Here's how the part is built. I have some questions about the finished solid (model axes, mm). Face numbers are marked on the shaded views. A direction names the side the tool comes from. Round coordinates to 2 decimals unless told otherwise and drop trailing zeros. Write each loop counter-clockwise with the first axis right and the second up, starting at its lowest first coordinate (ties: lowest second). Pieces come first, ordered by that corner, then holes. Notation, with made-up numbers: M 31.5,54 L 39.5,54 A16 ccw 39.5,78 Z; hole C 28,4 d4. An arc over 180 degrees is marked long. Use a Markdown table: item, result. Add a question column.
```python
from build123d import *

# Parameters (mm, degrees)
SKETCH1_R           = 1.5
BOSS_EXTRUDE1_DEPTH = 3


with BuildPart() as part:
    # Sketch1 → Boss-Extrude1 (new body)
    with BuildSketch(Plane.XY):
        with BuildLine():
            Line((0, 7), (0, 12))
            Line((0, 12), (3, 12))
            Line((3, 12), (3, 16))
            Line((3, 16), (0, 16))
            Line((0, 16), (0, 21))
            Line((0, 21), (3, 21))
            Line((3, 21), (3, 25))
            Line((3, 25), (0, 25))
            Line((0, 25), (0, 30))
            Line((0, 30), (3, 30))
            Line((3, 30), (3, 34))
            Line((3, 34), (0, 34))
            Line((0, 34), (0, 39))
            Line((0, 39), (3, 39))
            Line((3, 39), (3, 43))
            Line((3, 43), (0, 43))
            Line((0, 43), (0, 48))
            Line((0, 48), (3, 48))
            Line((3, 48), (3, 52))
            Line((3, 52), (0, 52))
            Line((0, 52), (0, 57))
            Line((0, 57), (3, 57))
            Line((3, 57), (3, 61))
            Line((3, 61), (0, 61))
            Line((0, 61), (0, 66))
            Line((0, 66), (3, 66))
            Line((3, 66), (3, 70))
            Line((3, 70), (0, 70))
            Line((0, 70), (0, 75))
            Line((0, 75), (3, 75))
            Line((3, 75), (3, 79))
            Line((3, 79), (0, 79))
            Line((0, 79), (0, 84))
            Line((0, 84), (2, 84))
            ThreePointArc((2, 84), (4.121320344, 83.121320344), (5, 81))
            Line((5, 81), (5, 59.197256694))
            ThreePointArc((5, 59.197256694), (5.006464082, 59.000425028), (5.02582847, 58.804441586))
            Line((5.02582847, 58.804441586), (12, 6))
            Line((12, 6), (12, 4))
            ThreePointArc((12, 4), (10.828427125, 1.171572875), (8, 0))
            Line((8, 0), (0, 0))
            Line((0, 0), (0, 3))
            Line((0, 3), (3, 3))
            Line((3, 3), (3, 7))
            Line((3, 7), (0, 7))
        make_face()
        with Locations((8, 5)):
            Circle(SKETCH1_R, mode=Mode.SUBTRACT)
    extrude(amount=BOSS_EXTRUDE1_DEPTH)


solid = part.part
```
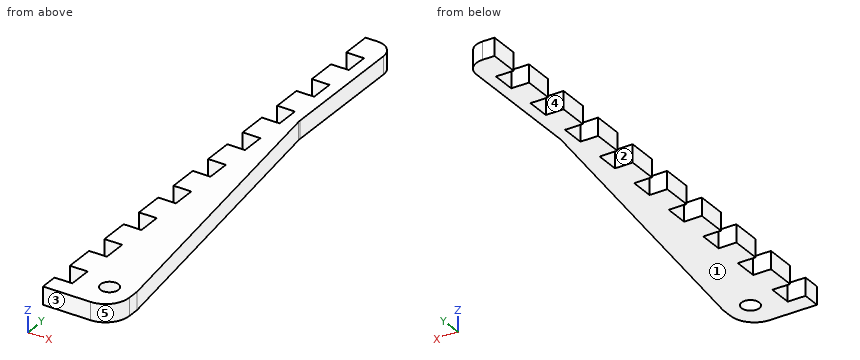
Item 1: If we mould it in two halves opening along Y, with no side actions, what happens to the marked faces 1, 2 and 3? For each: +Y half, -Y half, draft (parallel to the pull), parting line (faces both ways), or undercut.
Item 2: Imagine slicing it at B-B on x = 8.75. List the corners of the cut face in (y, z) for me.
Item 3: Imagine slicing it at A-A on y = 5. List the corners of the cut face in (x, z) for me, plus the area to 3 significant figures.
Item 4: I need wall thicknesses on probe 1 along X at (y, z) = (59, 2.45); probe 2 along X at (y, z) = (4.5, 0.6); probe 3 along X at (y, z) = (43.5, 2.85). Which ranges of each line are inside material? Lowest first, please. Write a range as from..to.
Item 5: On a 3-axis mill with a long thin cutter (end or side, diameter ignored), from which of +Z, -Z, +X, -X, +Y, -Y can I reach the whole of each face in a straight line? I mean the marked faces 4 and 5. Say none if no direction works.
Item 6: Imagine slicing it at C-C on y = 28. List the corners of the cut face in (x, z) for me.
Item 7: Imagine slicing it at D-D on y = 54. List the corners of the cut face in (x, z) for me, plus the area to 3 significant figures.
Item 8: For pin 1 Ø1.5 at (y, z) = (23.5, 1) entering from -X; pin 2 Ø1 at (y, z) = (16.5, 1.5) entering from +X; pin 3 Ø0.9 at (y, z) = (69.5, 1) entering from +X, each with a flat end and sliding along its axis, tell me the tip position at first contact or that it passes through.
The answers:
| question | item | result |
|---|---|---|
| 1 | face 1 | draft |
| 1 | face 2 | undercut |
| 1 | face 3 | -Y half |
| 2 | outline | M 0.07,0 L 3.7,0 L 3.7,3 L 0.07,3 Z; M 6.3,0 L 30.61,0 L 30.61,3 L 6.3,3 Z |
| 3 | outline | M 3,0 L 6.5,0 L 6.5,3 L 3,3 Z; M 9.5,0 L 12,0 L 12,3 L 9.5,3 Z |
| 3 | area | 18.0 mm² |
| 4 | probe 1 | 3..5.01 |
| 4 | probe 2 | 3..6.59, 9.41..12 |
| 4 | probe 3 | 0..7.05 |
| 5 | face 4 | +Z, -Z, -X |
| 5 | face 5 | +Z, -Z, +X, -Y |
| 6 | outline | M 0,0 L 9.09,0 L 9.09,3 L 0,3 Z |
| 7 | outline | M 0,0 L 5.66,0 L 5.66,3 L 0,3 Z |
| 7 | area | 17.0 mm² |
| 8 | pin 1 | x = 3 |
| 8 | pin 2 | x = 10.68 |
| 8 | pin 3 | x = 5 |
